Here's how the part is built. I have some questions about the finished solid (model axes, mm). Face numbers are marked on the shaded views. A direction names the side the tool comes from. Round coordinates to 2 decimals unless told otherwise and drop trailing zeros. Write each loop counter-clockwise with the first axis right and the second up, starting at its lowest first coordinate (ties: lowest second). Pieces come first, ordered by that corner, then holes. Notation, with made-up numbers: (27, -18.75) - (81, -18.75) arc R11 ccw to (81, 1.25) - close; hole circle Ø7 at (-16, -3.75). An arc over 180 degrees is marked (long way). One line per question, with ' | ' between items. Start each with the question number.
(1) Imagine slicing it at B-B (z = 9.5). Write out the boundary of the cut face in (x, y), plus the area to 3 significant figures.
(2) If I drill on L1, parallel to Z at x = 23.35, y = 0; L2, parallel to Y at x = 0.5, z = 14; L3, parallel to X at y = -13, z = 32.5, over which ranges is the centre line in solid material (lowest first)?
(3) For the marked faces 1, 2 and 3, which set-ups out of +Z, -Z, +X, -X, +Y, -Y let a thin tool reach every point of the face, with its end or its side?
(4) Will these pins go through, and if not, where does the flat tip stop? pin 1 (1.6 mm diameter, centred on x = 13, z = -1.5, fed in from +Y); pin 2 (12 mm diameter, centred on x = -16, z = 1.5, fed in from -Y); pin 3 (0.6 mm diameter, centred on x = 10, z = 33, fed in from -Y); pin 4 (1 mm diameter, centred on x = 11.5, z = 33, fed in from +Y).
(5) Imagine slicing it at A-A (y = 12). Write out the boundary of the cut face in (x, z), plus the area to 3 significant figures.
(6) Imagine slicing it at C-C (y = -9). Write out the boundary of the cut face in (x, z), plus the area to 3 significant figures.
(7) Thinking about a two-plate mould opening in Y: for the marked faces 4, 5 and 6, which applies, pulls with the +Y half, pulls with the -Y half, needs draft (parallel to the pull), parting line crosses it, or undercut?
from build123d import *

# Parameters (mm, degrees)
SKETCH_W        = 53
SKETCH_H        = 37.5
SKETCH_W_2      = 49
SKETCH_H_2      = 33.5
PAD_DEPTH       = 32
SKETCH001_W     = 53
SKETCH001_H     = 37.5
PAD001_DEPTH    = 2
SKETCH002_W     = 53
SKETCH002_H     = 37.5
PAD002_DEPTH    = 2
SKETCH003_W     = 33.5
SKETCH003_H     = 32
POCKET_DEPTH    = 2
SKETCH004_W     = 10
SKETCH004_H     = 5.75
SKETCH004_W_2   = 12.5
SKETCH004_W_3   = 9.9999999999
POCKET001_DEPTH = 5
SKETCH005_W     = 51
SKETCH005_H     = 1.8
SKETCH005_H_2   = 1.5
PAD003_DEPTH    = 33.5
SKETCH006_W     = 30.5
SKETCH006_H     = 9
POCKET002_DEPTH = 51
SKETCH007_W     = 17.616245
SKETCH007_H     = 6
PAD004_DEPTH    = 5
SKETCH008_R     = 0.8
POCKET003_DEPTH = 5
SKETCH009_W     = 17.616245
SKETCH009_H     = 6
PAD005_DEPTH    = 3.5
SKETCH010_R     = 0.8
POCKET004_DEPTH = 6
CHAMFER_SIZE    = 3.499
CHAMFER001_SIZE = 4.99
FILLET_R        = 1.99
SKETCH012_W     = 53
SKETCH012_H     = 4
PAD006_DEPTH    = 6
FILLET001_R     = 5
SKETCH013_W     = 6
SKETCH013_H     = 5
POCKET005_DEPTH = 20
SKETCH014_W     = 10
SKETCH014_H     = 18
POCKET006_DEPTH = 5


with BuildPart() as part:
    # Sketch → Pad (new body)
    with BuildSketch(Plane.XY):
        Rectangle(SKETCH_W, SKETCH_H)
        Rectangle(SKETCH_W_2, SKETCH_H_2, mode=Mode.SUBTRACT)
    extrude(amount=PAD_DEPTH)

    # Sketch001 (on Face10 of Pad) → Pad001 (join)
    with BuildSketch(Plane.XY.offset(32)):
        Rectangle(SKETCH001_W, SKETCH001_H)
    extrude(amount=PAD001_DEPTH)

    # Sketch002 (on Face4 of Pad001) → Pad002 (join)
    with BuildSketch(Plane(origin=(0, 0, 0), x_dir=(1, 0, 0), z_dir=(0, 0, -1))):
        Rectangle(SKETCH002_W, SKETCH002_H)
    extrude(amount=PAD002_DEPTH)

    # Sketch003 (on Face3 of Pad002) → Pocket (cut)
    with BuildSketch(Plane.YZ.offset(26.5)):
        with Locations((0, 16)):
            Rectangle(SKETCH003_W, SKETCH003_H)
    extrude(amount=-POCKET_DEPTH, mode=Mode.SUBTRACT)

    # Sketch004 (on Face13 of Pocket) → Pocket001 (cut)
    with BuildSketch(Plane.XY.offset(34)):
        with Locations((-16.4, -10.975)):
            Rectangle(SKETCH004_W, SKETCH004_H)
        with Locations((-2.5, -10.975)):
            Rectangle(SKETCH004_W_2, SKETCH004_H)
        with Locations((11.45, -10.975)):
            Rectangle(SKETCH004_W_3, SKETCH004_H)
    extrude(amount=-POCKET001_DEPTH, mode=Mode.SUBTRACT)

    # Sketch005 (on Face36 of Pocket001) → Pad003 (join)
    with BuildSketch(Plane(origin=(0, -16.75, 0), x_dir=(-1, 0, 0), z_dir=(0, 1, 0))):
        with Locations((-1, 22.25)):
            Rectangle(SKETCH005_W, SKETCH005_H)
        with Locations((-1, 26)):
            Rectangle(SKETCH005_W, SKETCH005_H_2)
        with Locations((-1, 18.5)):
            Rectangle(SKETCH005_W, SKETCH005_H_2)
    extrude(amount=PAD003_DEPTH)

    # Sketch006 (on Face11 of Pad003) → Pocket002 (cut)
    with BuildSketch(Plane.YZ.offset(26.5)):
        with Locations((0, 22.25)):
            Rectangle(SKETCH006_W, SKETCH006_H)
    extrude(amount=-POCKET002_DEPTH, mode=Mode.SUBTRACT)

    # Sketch007 (on Face57 of Pocket002) → Pad004 (join)
    with BuildSketch(Plane.XY):
        with Locations((17.6918775, 0)):
            Rectangle(SKETCH007_W, SKETCH007_H)
    extrude(amount=PAD004_DEPTH)

    # Sketch008 (on Face24 of Pad004) → Pocket003 (cut)
    with BuildSketch(Plane.YZ.offset(26.5)):
        with Locations((0, 2.5)):
            Circle(SKETCH008_R)
    extrude(amount=-POCKET003_DEPTH, mode=Mode.SUBTRACT)

    # Sketch009 (on Face65 of Pocket003) → Pad005 (join)
    with BuildSketch(Plane(origin=(0, 0, 32), x_dir=(1, 0, 0), z_dir=(0, 0, -1))):
        with Locations((17.6918775, 0)):
            Rectangle(SKETCH009_W, SKETCH009_H)
    extrude(amount=PAD005_DEPTH)

    # Sketch010 (on Face41 of Pad005) → Pocket004 (cut)
    with BuildSketch(Plane.YZ.offset(26.5)):
        with Locations((0, 30.25)):
            Circle(SKETCH010_R)
    extrude(amount=-POCKET004_DEPTH, mode=Mode.SUBTRACT)

    # Chamfer
    chamfer_edges = [part.edges().sort_by_distance(p)[0] for p in [
        (8.883755, 0, 28.5),
    ]]
    chamfer(chamfer_edges, length=CHAMFER_SIZE)

    # Chamfer001
    chamfer001_edges = [part.edges().sort_by_distance(p)[0] for p in [
        (8.883755, 0, 5),
    ]]
    chamfer(chamfer001_edges, length=CHAMFER001_SIZE)

    # Fillet
    fillet_edges = [part.edges().sort_by_distance(p)[0] for p in [
        (0, -18.75, 34),
        (0, 18.75, 34),
        (0, 18.75, -2),
        (0, -18.75, -2),
    ]]
    fillet(fillet_edges, radius=FILLET_R)

    # Sketch012 → Pad006 (join)
    with BuildSketch(Plane.XZ.offset(18.75)):
        with Locations((0, 23.8)):
            Rectangle(SKETCH012_W, SKETCH012_H)
        with Locations((0, 8.5)):
            Rectangle(SKETCH012_W, SKETCH012_H)
    extrude(amount=PAD006_DEPTH)

    # Fillet001
    fillet001_edges = [part.edges().sort_by_distance(p)[0] for p in [
        (0, -18.75, 6.5),
        (0, -18.75, 25.8),
    ]]
    fillet(fillet001_edges, radius=FILLET001_R)

    # Sketch013 (on Face26 of Fillet001) → Pocket005 (cut)
    with BuildSketch(Plane.YZ.offset(26.5)):
        with Locations((0, 2.5)):
            Rectangle(SKETCH013_W, SKETCH013_H)
    extrude(amount=-POCKET005_DEPTH, mode=Mode.SUBTRACT)

    # Sketch014 (on Face23 of Pocket005) → Pocket006 (cut)
    with BuildSketch(Plane(origin=(0, 0, -2), x_dir=(1, 0, 0), z_dir=(0, 0, -1))):
        with Locations((12.5, -5.75)):
            Rectangle(SKETCH014_W, SKETCH014_H)
    extrude(amount=-POCKET006_DEPTH, mode=Mode.SUBTRACT)


solid = part.part
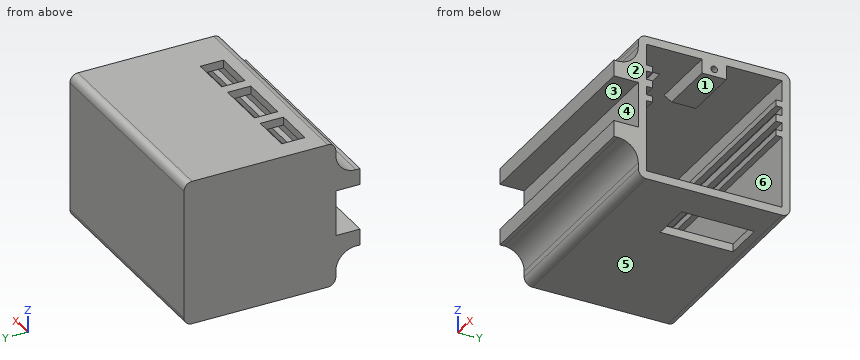
Check sheet entries:
1) outline: (-26.5, -24.75) - (26.5, -24.75) - (26.5, -16.75) - (-24.5, -16.75) - (-24.5, 16.75) - (26.5, 16.75) - (26.5, 18.75) - (-26.5, 18.75) - close | area: 597 mm^2
2) L1: -2 to 0, 28.5 to 29.45, 31.05 to 34 | L2: -18.75 to -16.75, 16.75 to 18.75 | L3: -26.5 to -21.4, -11.4 to -8.75, 3.75 to 6.45, 16.45 to 26.5
3) face 1: +X | face 2: +Z, -Z, +X, +Y, -Y | face 3: +X, -X, -Y
4) pin 1: y = 18.63 | pin 2: y = -24.75 | pin 3: y = -18.63 | pin 4: y = 18.69
5) outline: (-26.5, -2) - (7.5, -2) - (7.5, 0) - (-24.5, 0) - (-24.5, 32) - (26.5, 32) - (26.5, 34) - (-26.5, 34) - close; (17.5, -2) - (26.5, -2) - (26.5, 0) - (17.5, 0) - close | area: 256 mm^2
6) outline: (-26.5, -2) - (26.5, -2) - (26.5, 0) - (-24.5, 0) - (-24.5, 32) - (-21.4, 32) - (-21.4, 34) - (-26.5, 34) - close; (-11.4, 32) - (-8.75, 32) - (-8.75, 34) - (-11.4, 34) - close; (3.75, 32) - (6.45, 32) - (6.45, 34) - (3.75, 34) - close; (16.45, 32) - (26.5, 32) - (26.5, 34) - (16.45, 34) - close | area: 211 mm^2
7) face 4: pulls with the -Y half | face 5: needs draft | face 6: undercut
